Source: CAD feature listing. Evaluate the final solid. Frame: model axes, mm. A direction names the side the tool comes from. Give positions to 0.01 mm unless a question says otherwise; leave off trailing zeros. Loops run counter-clockwise (first coordinate to the right, second up) from the corner with the lowest first, then second, coordinate; pieces in that order, holes last. Notation, with made-up numbers: (-21.5, -15.5) -> (2.5, -15.5) arc R25 cw to (2.5, 2.5) -> close; hole circle Ø5 at (88, 39.25). An arc over 180 degrees is marked (long way). Return JSON: item names as keys, results as strings. Group by question number.
(1) Access query for faces 4 (the face through (-7.5, 0, 2)), 5 (the face through (-7, 0, 5)), 6 (the face through (6.45, 0, 6)). Directions: +Z, -Z, +X, -X, +Y, -Y. A direction counts if a zero-diameter tool reaches every point of the face in a straight line with its end or side. Return the directions, or none.
(2) Cut plane A-A on x = 0. Return loops of the section in (y, z).
(3) Pin query (flat end, axial travel): pin 1 (1 mm diameter, centred on y = 3, z = 6, fed in from -X); pin 2 (0.8 mm diameter, centred on x = -7, y = 2.5, fed in from -Z); pin 3 (0.6 mm diameter, centred on y = 0.5, z = 6, fed in from +X). Return the tip coordinate at first contact, or that it passes through.
(4) Cut plane C-C on z = 4.75. Return loops of the section in (x, y).
(5) Ray query, line 1 (Y direction, x = 0, z = 1.75); line 2 (Z direction, x = 6.75, y = 1.25); line 3 (Y direction, x = 2.5, z = 2.25). Return the intervals inside material, ascending. Write a range as from..to.
(6) Draft query along Z for faces 1 (the face through (7, 0, 5)), 2 (the face through (0, -6, 4)), 3 (the face through (0, -3, 8)). Return one class per face: released by +Z, released by -Z, zero draft, split by the parting line, or undercut.
(7) Cut plane D-D on y = -3.5. Return loops of the section in (x, z).
(8) Cut plane B-B on y = 0.5. Return loops of the section in (x, z).
```python
from build123d import *

# Parameters (mm, degrees)
ESQUISSE1_W             = 15
ESQUISSE1_H             = 12
BOSS_EXTRU_1_DEPTH      = 5
ESQUISSE2_W             = 12.95
ESQUISSE2_H             = 12
BOSS_EXTRU_2_DEPTH      = 2.05
ESQUISSE3_W             = 15
ESQUISSE3_H             = 12
BOSS_EXTRU_3_DEPTH      = 0.95
ESQUISSE4_R             = 3.05
ENL_V_MAT_EXTRU_1_DEPTH = 8


with BuildPart() as part:
    # Esquisse1 → Boss.-Extru.1 (new body)
    with BuildSketch(Plane.XY):
        Rectangle(ESQUISSE1_W, ESQUISSE1_H)
    extrude(amount=BOSS_EXTRU_1_DEPTH)

    # Esquisse2 → Boss.-Extru.2 (add)
    with BuildSketch(Plane.XY.offset(5)):
        with Locations((-0.025, 0)):
            Rectangle(ESQUISSE2_W, ESQUISSE2_H)
    extrude(amount=BOSS_EXTRU_2_DEPTH)

    # Esquisse3 → Boss.-Extru.3 (add)
    with BuildSketch(Plane.XY.offset(7.05)):
        Rectangle(ESQUISSE3_W, ESQUISSE3_H)
    extrude(amount=BOSS_EXTRU_3_DEPTH)

    # Esquisse4 → Enlèv. mat.-Extru.1 (cut)
    with BuildSketch(Plane.XY.offset(8)):
        with Locations((0, 0.5)):
            Circle(ESQUISSE4_R)
    extrude(amount=-ENL_V_MAT_EXTRU_1_DEPTH, mode=Mode.SUBTRACT)


solid = part.part
```
Answers:
{
 "1": {"face 4": "+Z, -Z, -X, +Y, -Y", "face 5": "-X, +Y, -Y", "face 6": "+X, +Y, -Y"},
 "2": {"outline": "(-6, 0) -> (-2.55, 0) -> (-2.55, 8) -> (-6, 8) -> close; (3.55, 0) -> (6, 0) -> (6, 8) -> (3.55, 8) -> close"},
 "3": {"pin 1": "x = -6.5", "pin 2": "z = 0", "pin 3": "x = 6.45"},
 "4": {"outline": "(-7.5, -6) -> (7.5, -6) -> (7.5, 6) -> (-7.5, 6) -> close; hole circle Ø6.1 at (0, 0.5)"},
 "5": {"line 1": "-6..-2.55, 3.55..6", "line 2": "0..5, 7.05..8", "line 3": "-6..-1.25, 2.25..6"},
 "6": {"face 1": "undercut", "face 2": "zero draft", "face 3": "released by +Z"},
 "7": {"outline": "(-7.5, 0) -> (7.5, 0) -> (7.5, 5) -> (6.45, 5) -> (6.45, 7.05) -> (7.5, 7.05) -> (7.5, 8) -> (-7.5, 8) -> (-7.5, 7.05) -> (-6.5, 7.05) -> (-6.5, 5) -> (-7.5, 5) -> close"},
 "8": {"outline": "(-7.5, 0) -> (-3.05, 0) -> (-3.05, 8) -> (-7.5, 8) -> (-7.5, 7.05) -> (-6.5, 7.05) -> (-6.5, 5) -> (-7.5, 5) -> close; (3.05, 0) -> (7.5, 0) -> (7.5, 5) -> (6.45, 5) -> (6.45, 7.05) -> (7.5, 7.05) -> (7.5, 8) -> (3.05, 8) -> close"}
}
